Could you check a few things on this model? Use its own coordinates, in mm. Face numbers are marked on the shaded views. A direction names the side the tool comes from. Give positions to 0.01 mm unless a question says otherwise; leave off trailing zeros. Loops run counter-clockwise (first coordinate to the right, second up) from the corner with the lowest first, then second, coordinate; pieces in that order, holes last.
1. For P1, Ø6, axis at x = -32, y = -1.5, coming from the +Z side; P2, Ø1.8, axis at x = -6.5, z = 13, coming from the +Y side; P3, Ø2.5, axis at x = -33.34, y = -141.47, coming from the +Z side, each with a flat end and sliding along its axis, tell me the tip position at first contact or that it passes through.
2. Imagine slicing it at A-A (z = 9.5). Count the separate pieces of the cut face and the enclosed holes in it, plus the area to 3 significant figures.
3. Imagine slicing it at B-B (y = -120). List the corners of the cut face in (x, z) for me (3 decimals), plus the area to 4 significant figures.
4. I need wall thicknesses on line 1 along X through (y, z) = (-141.47, 4) (3 decimals); line 2 along X through (y, z) = (-94.5, 13) (3 decimals); line 3 along X through (y, z) = (-122, 2.5) (3 decimals). Which ranges of each line are inside material? Lowest first, please.
5. For the marked faces 1 and 2, which set-ups out of +Z, -Z, +X, -X, +Y, -Y let a thin tool reach every point of the face, with its end or its side?
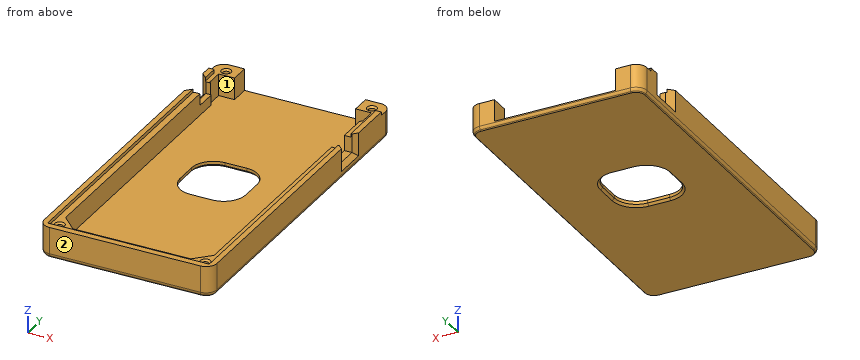
```python
from build123d import *

# Parameters (mm, degrees)
SKETCH_W        = 79.03
SKETCH_H        = 156.85
PAD_DEPTH       = 14
POCKET_DEPTH    = 11.6
PAD001_DEPTH    = 10
SKETCH003_R     = 1.45
POCKET001_DEPTH = 12
FILLET_R        = 5
CHAMFER_SIZE    = 1
FILLET001_R     = 2
CHAMFER001_SIZE = 0.8
SKETCH004_W     = 12.65
SKETCH004_H     = 11
POCKET002_DEPTH = 8.6
SKETCH005_W     = 11.08
SKETCH005_H     = 10
POCKET003_DEPTH = 7
SKETCH006_R     = 1.45
POCKET004_DEPTH = 12
SKETCH007_W     = 92.15
SKETCH007_H     = 16.7
POCKET005_DEPTH = 1.6
CHAMFER002_SIZE = 0.8
SKETCH008_W     = 30
SKETCH008_H     = 30
POCKET006_DEPTH = 2.401
FILLET002_R     = 10
CHAMFER003_SIZE = 1
CHAMFER004_SIZE = 3
CHAMFER005_SIZE = 2


with BuildPart() as part:
    # Sketch → Pad (new body)
    with BuildSketch(Plane.XY):
        with Locations((0, -69.725)):
            Rectangle(SKETCH_W, SKETCH_H)
    extrude(amount=PAD_DEPTH)

    # Sketch001 (on Face6 of Pad) → Pocket (cut)
    with BuildSketch(Plane.XY.offset(14)):
        Polygon((-37.015, -145.15), (37.015, -145.15), (37.015, 0), (27.7, 0), (27.7, 8.7), (-27.7, 8.7), (-27.7, 0), (-37.015, 0), align=None)
    extrude(amount=-POCKET_DEPTH, mode=Mode.SUBTRACT)

    # Sketch002 (on Face6 of Pocket) → Pad001 (join)
    with BuildSketch(Plane.XY.offset(2.4)):
        Polygon((-35.015, 0), (-35.015, -7.5), (-34.015, -8.5), (-34.015, -135.15), (-27.015, -142.15), (27.015, -142.15), (34.015, -135.15), (34.015, -8.5), (35.015, -7.5), (35.015, 0), (37.015, 0), (37.015, -145.15), (-37.015, -145.15), (-37.015, 0), align=None)
    extrude(amount=PAD001_DEPTH)

    # Sketch003 (on Face24 of Pad001) → Pocket001 (cut)
    with BuildSketch(Plane.XY.offset(12.4)):
        with Locations((-33.34, -141.47)):
            Circle(SKETCH003_R)
        with Locations((33.34, -141.47)):
            Circle(SKETCH003_R)
    extrude(amount=-POCKET001_DEPTH, mode=Mode.SUBTRACT)

    # Fillet
    fillet_edges = [part.edges().sort_by_distance(p)[0] for p in [
        (39.515, 8.7, 7),
        (39.515, -148.15, 7),
        (-39.515, 8.7, 7),
        (-39.515, -148.15, 7),
    ]]
    fillet(fillet_edges, radius=FILLET_R)

    # Chamfer
    chamfer_edges = [part.edges().sort_by_distance(p)[0] for p in [
        (-38.050534, 7.235534, 0),
    ]]
    chamfer(chamfer_edges, length=CHAMFER_SIZE)

    # Fillet001
    fillet001_edges = [part.edges().sort_by_distance(p)[0] for p in [
        (-38.050534, 7.235534, 1),
    ]]
    fillet(fillet001_edges, radius=FILLET001_R)

    # Chamfer001
    chamfer001_edges = [part.edges().sort_by_distance(p)[0] for p in [
        (-34.79, -141.47, 12.4),
        (31.89, -141.47, 12.4),
    ]]
    chamfer(chamfer001_edges, length=CHAMFER001_SIZE)

    # Sketch004 (on Face20 of Chamfer001) → Pocket002 (cut)
    with BuildSketch(Plane.XY.offset(14)):
        with Locations((37.485, -27.31)):
            Rectangle(SKETCH004_W, SKETCH004_H)
    extrude(amount=-POCKET002_DEPTH, mode=Mode.SUBTRACT)

    # Sketch005 (on Face16 of Pocket002) → Pocket003 (cut)
    with BuildSketch(Plane.XY.offset(14)):
        with Locations((-36.33, -13.2)):
            Rectangle(SKETCH005_W, SKETCH005_H)
    extrude(amount=-POCKET003_DEPTH, mode=Mode.SUBTRACT)

    # Sketch006 → Pocket004 (cut)
    with BuildSketch(Plane.XY.offset(14)):
        with Locations((-33.34, 3.5)):
            Circle(SKETCH006_R)
        with Locations((33.34, 3.5)):
            Circle(SKETCH006_R)
    extrude(amount=-POCKET004_DEPTH, mode=Mode.SUBTRACT)

    # Sketch007 (on Face7 of Pocket004) → Pocket005 (cut)
    with BuildSketch(Plane.XY.offset(14)):
        with Locations((0, 8.35)):
            Rectangle(SKETCH007_W, SKETCH007_H)
    extrude(amount=-POCKET005_DEPTH, mode=Mode.SUBTRACT)

    # Chamfer002
    chamfer002_edges = [part.edges().sort_by_distance(p)[0] for p in [
        (31.89, 3.5, 12.4),
        (-34.79, 3.5, 12.4),
    ]]
    chamfer(chamfer002_edges, length=CHAMFER002_SIZE)

    # Sketch008 (on Face16 of Chamfer002) → Pocket006 (cut, through all)
    with BuildSketch(Plane.XY.offset(2.4)):
        with Locations((-1.59, -63.5)):
            Rectangle(SKETCH008_W, SKETCH008_H)
    extrude(amount=-POCKET006_DEPTH, mode=Mode.SUBTRACT)

    # Fillet002
    fillet002_edges = [part.edges().sort_by_distance(p)[0] for p in [
        (-16.59, -48.5, 1.2),
        (13.41, -48.5, 1.2),
        (13.41, -78.5, 1.2),
        (-16.59, -78.5, 1.2),
    ]]
    fillet(fillet002_edges, radius=FILLET002_R)

    # Chamfer003
    chamfer003_edges = [part.edges().sort_by_distance(p)[0] for p in [
        (-13.661068, -75.571068, 0),
    ]]
    chamfer(chamfer003_edges, length=CHAMFER003_SIZE)

    # Chamfer004
    chamfer004_edges = [part.edges().sort_by_distance(p)[0] for p in [
        (-39.515, -18.2, 10.5),
        (-39.515, -13.2, 7),
        (-39.515, -8.2, 10.5),
    ]]
    chamfer(chamfer004_edges, length=CHAMFER004_SIZE)

    # Chamfer005
    chamfer005_edges = [part.edges().sort_by_distance(p)[0] for p in [
        (39.515, -32.81, 9.7),
        (39.515, -27.31, 5.4),
        (39.515, -21.81, 9.7),
    ]]
    chamfer(chamfer005_edges, length=CHAMFER005_SIZE)


solid = part.part
```
Derived:
1. P1: stops at z = 12.4
1. P2: stops at y = -142.15
1. P3: stops at z = 0.4
2. separate pieces: 3
2. enclosed holes: 4
2. area: 2,100 mm2
3. outline: (-39.515, 1.828) arc R2 ccw to (-38.929, 0.414) - (-38.515, 0) - (38.515, 0) - (38.929, 0.414) arc R2 ccw to (39.515, 1.828) - (39.515, 14) - (37.015, 14) - (37.015, 12.4) - (34.015, 12.4) - (34.015, 2.4) - (-34.015, 2.4) - (-34.015, 12.4) - (-37.015, 12.4) - (-37.015, 14) - (-39.515, 14) - close
3. area: 306.5 mm2
4. line 1: x = -39.515 to -34.79, -31.89 to -27.695, 27.695 to 31.89, 34.79 to 39.515
4. line 2: x = -39.515 to -37.015, 37.015 to 39.515
4. line 3: x = -39.515 to -34.015, 34.015 to 39.515
5. face 1: +Z
5. face 2: +Z, -Z, +X, -X, -Y
